Read the model definition and answer for the solid it produces. Units are mm, in the model's axes. Coordinates: 2 decimals unless noted, no trailing zeros. Loops run counter-clockwise (first coordinate to the right, second up) from the corner with the lowest first, then second, coordinate; pieces in that order, holes last.
from build123d import *

# Parameters (mm, degrees)
SKETCH010_R  = 3.9
SKETCH010_W  = 17.8
SKETCH010_H  = 4.8
PAD010_DEPTH = 5


with BuildPart() as part:
    # Sketch010 → Pad010 (new body)
    with BuildSketch(Plane.XY):
        Polygon((-10.1, 160.1), (-20.2, 160.1), (-31.1, 42.945185), (-31.1, 20.1), (-33.2255, 20.1), (-47.2, -130.1), (-33.6, -130.1), (-33.6, -155.2), (-13.4, -155.2), (-13.4, -130.1), (13.4, -130.1), (13.4, -155.2), (33.6, -155.2), (33.6, -130.1), (47.2, -130.1), (33.2255, 20.1), (31.1, 20.1), (31.1, 42.945185), (20.2, 160.1), (10.1, 160.1), (10.1, 185.2), (-10.1, 185.2), align=None)
        with Locations((0, -100)):
            Circle(SKETCH010_R, mode=Mode.SUBTRACT)
        with Locations((0, 100)):
            Circle(SKETCH010_R, mode=Mode.SUBTRACT)
        with Locations((0, 117.5)):
            Rectangle(SKETCH010_W, SKETCH010_H, mode=Mode.SUBTRACT)
        with Locations((0, 82.5)):
            Rectangle(SKETCH010_W, SKETCH010_H, mode=Mode.SUBTRACT)
        with Locations((0, -117.5)):
            Rectangle(SKETCH010_W, SKETCH010_H, mode=Mode.SUBTRACT)
        with Locations((0, -82.5)):
            Rectangle(SKETCH010_W, SKETCH010_H, mode=Mode.SUBTRACT)
    extrude(amount=PAD010_DEPTH)


solid = part.part
Q1. A cutting plane is placed at A-A (x = 0). Give the vertices of the cut face in (y, z).
Findings below:
outline: (-130.1, 0) - (-119.9, 0) - (-119.9, 5) - (-130.1, 5) - close; (-115.1, 0) - (-103.9, 0) - (-103.9, 5) - (-115.1, 5) - close; (-96.1, 0) - (-84.9, 0) - (-84.9, 5) - (-96.1, 5) - close; (-80.1, 0) - (80.1, 0) - (80.1, 5) - (-80.1, 5) - close; (84.9, 0) - (96.1, 0) - (96.1, 5) - (84.9, 5) - close; (103.9, 0) - (115.1, 0) - (115.1, 5) - (103.9, 5) - close; (119.9, 0) - (185.2, 0) - (185.2, 5) - (119.9, 5) - close
Q2. A cutting plane is placed at C-C (z = 4.05). Count the separate pieces of the cut face and the enclosed holes in it, then the cut area to 3 significant figures.
Findings below:
separate pieces: 1
enclosed holes: 6
area: 20,600 mm2
Q3. Flat-ended cylindrical pins translate along their axes: pin 1 Ø6 at (x, y) = (0, -100) entering from +Z; pin 2 Ø2.5 at (x, z) = (-0.5, 2.5) entering from -Y; pin 3 Ø1.4 at (y, z) = (-116.5, 2) entering from +X; pin 4 Ø2.5 at (x, z) = (13.5, 3.5) entering from +Y. Find the tip coordinate at first contact, or state that the pin passes through.
Findings below:
pin 1: passes through
pin 2: stops at y = -130.1
pin 3: stops at x = 46
pin 4: stops at y = 160.1
Q4. Straight lines are drawn through the part: probe 1 along Y at (x, z) = (4, 3.6); probe 2 along Y at (x, z) = (-14, 1.7); probe 3 along X at (y, z) = (150, 3.1). For each, find the intervals that lie inside material, in ascending order.
Findings below:
probe 1: y = -130.1 to -119.9, -115.1 to -84.9, -80.1 to 80.1, 84.9 to 115.1, 119.9 to 185.2
probe 2: y = -155.2 to 160.1
probe 3: x = -21.14 to 21.14
Q5. A cutting plane is placed at B-B (y = -100). Give the vertices of the cut face in (x, z).
Findings below:
outline: (-44.4, 0) - (-3.9, 0) - (-3.9, 5) - (-44.4, 5) - close; (3.9, 0) - (44.4, 0) - (44.4, 5) - (3.9, 5) - close
Q6. Determine the mould class of faces 1 (the face through (-1, -20, 0)), 2 (the face through (40.31, -56.05, 2.46)), 3 (the face through (-0.845, 96.193, 2.465)) for opening direction X: +X half, -X half, draft (parallel to the pull), parting line (faces both ways), or undercut.
Findings below:
face 1: draft
face 2: +X half
face 3: undercut
Q7. A cutting plane is placed at D-D (y = 100). Give the vertices of the cut face in (x, z), then the cut area to 3 significant figures.
Findings below:
outline: (-25.79, 0) - (-3.9, 0) - (-3.9, 5) - (-25.79, 5) - close; (3.9, 0) - (25.79, 0) - (25.79, 5) - (3.9, 5) - close
area: 219 mm2
